```python
from build123d import *

# Parameters (mm, degrees)
F0_W         = 27.2
F0_H         = 2.5
F0_W_2       = 2.5
F0_H_2       = 33.7
F1_DEPTH     = 3
F2_R         = 2
F3_DEPTH     = 2
F4_W         = 2.5
F4_H         = 2.5
F5_DEPTH     = 1
F6_T1_DEPTH  = 9
F6_S5_W      = 2
F6_S5_H      = 2
F6_T6_DEPTH  = 2
F6_S11_W     = 2
F6_S11_H     = 2
F6_T12_DEPTH = 2
F6_S17_W     = 2
F6_S17_H     = 2
F6_T18_DEPTH = 2
F6_S23_W     = 2
F6_S23_H     = 2
F6_T24_DEPTH = 2


# Not quite as in the source:
# - a fillet or chamfer that OpenCascade refuses, or shapes differently, is made with other operations: its cross-section is extruded or revolved along the edge and cut away or added


with BuildPart() as f1:
    # F0 (on Top) → F1 (new body)
    with BuildSketch(Plane.XY):
        with Locations((0.1669520199, 18.5940534235)):
            Rectangle(F0_W, F0_H)
        with Locations((-14.6830479801, 0.4940534235)):
            Rectangle(F0_W_2, F0_H_2)
        with Locations((-14.6830479801, 18.5940534235)):
            Rectangle(F0_W_2, F0_H)
        with Locations((-14.6830479801, -17.6059465765)):
            Rectangle(F0_W_2, F0_H)
        with Locations((0.1669520199, -17.6059465765)):
            Rectangle(F0_W, F0_H)
        with Locations((15.0169520199, -17.6059465765)):
            Rectangle(F0_W_2, F0_H)
        with Locations((15.0169520199, 0.4940534235)):
            Rectangle(F0_W_2, F0_H_2)
        with Locations((15.0169520199, 18.5940534235)):
            Rectangle(F0_W_2, F0_H)
    extrude(amount=F1_DEPTH)

    # F2
    f2_edges = [f1.edges().sort_by_distance(p)[0] for p in [
        (16.266952, 0.494053, 3),
        (0.166952, 19.844053, 3),
        (-15.933048, 0.494053, 3),
        (0.166952, -18.855947, 3),
    ]]
    fillet(f2_edges, radius=F2_R)

    # F0 (on Top) → F3 (join)
    with BuildSketch(Plane.XY):
        with Locations((-14.6830479801, -17.6059465765)):
            Rectangle(F0_W_2, F0_H)
        with Locations((15.0169520199, -17.6059465765)):
            Rectangle(F0_W_2, F0_H)
        with Locations((15.0169520199, 18.5940534235)):
            Rectangle(F0_W_2, F0_H)
        with Locations((-14.6830479801, 18.5940534235)):
            Rectangle(F0_W_2, F0_H)
    extrude(amount=-F3_DEPTH)

    # F4 (on face) → F5 (join)
    with BuildSketch(Plane(origin=(0, 0, -2), x_dir=(1, 0, 0), z_dir=(0, 0, -1))):
        Polygon((-13.4330479801, -19.8440534235), (16.2669520199, -19.8440534235), (16.2669520199, 18.8559465765), (-15.9330479801, 18.8559465765), (-15.9330479801, -17.3440534235), (-13.4330479801, -17.3440534235), align=None)
        with Locations((-14.6830479801, -18.5940534235)):
            Rectangle(F4_W, F4_H)
    extrude(amount=F5_DEPTH)

    # F6: fillet of radius 2 on 4 edges, made by hand

    # F6_s2 → F6_t1 (cut)
    with BuildSketch(Plane.XY.offset(-8)):
        with BuildLine():
            ThreePointArc((16.2669520199, 17.8440534235), (15.6811655823, 19.2582669858), (14.2669520199, 19.8440534235))
            Line((14.2669520199, 19.8440534235), (16.2669520199, 19.8440534235))
            Line((16.2669520199, 19.8440534235), (16.2669520199, 17.8440534235))
        make_face()
        with BuildLine():
            ThreePointArc((16.2669520199, -16.8559465765), (15.6811655823, -18.2701601389), (14.2669520199, -18.8559465765))
            Line((14.2669520199, -18.8559465765), (16.2669520199, -18.8559465765))
            Line((16.2669520199, -18.8559465765), (16.2669520199, -16.8559465765))
        make_face()
        with BuildLine():
            ThreePointArc((-15.9330479801, -16.8559465765), (-15.3472615424, -18.2701601389), (-13.9330479801, -18.8559465765))
            Line((-13.9330479801, -18.8559465765), (-15.9330479801, -18.8559465765))
            Line((-15.9330479801, -18.8559465765), (-15.9330479801, -16.8559465765))
        make_face()
        with BuildLine():
            ThreePointArc((-15.9330479801, 17.8440534235), (-15.3472615424, 19.2582669858), (-13.9330479801, 19.8440534235))
            Line((-13.9330479801, 19.8440534235), (-15.9330479801, 19.8440534235))
            Line((-15.9330479801, 19.8440534235), (-15.9330479801, 17.8440534235))
        make_face()
    extrude(amount=F6_T1_DEPTH, mode=Mode.SUBTRACT)


with BuildPart() as f6_tool4:
    # F6_s5 → F6_t6 (new body)
    with BuildSketch(Plane.YZ.offset(-13.9330479801)):
        with Locations((18.8440534235, 2)):
            Rectangle(F6_S5_W, F6_S5_H)
    extrude(amount=-F6_T6_DEPTH)

    # F6_s7 → F6_t8 (revolve, cut)
    with BuildSketch(Plane(origin=(-13.9330479801, 17.8440534235, 1), x_dir=(0, -0.7071067812, -0.7071067812), z_dir=(0, 0.7071067812, -0.7071067812))):
        with BuildLine():
            ThreePointArc((0, -2), (2, 0), (0, 2))
            Line((0, 2), (0, -2))
        make_face()
    revolve(axis=Axis((-13.9330479801, 17.8440534235, 1), (-1, 0, 0)), mode=Mode.SUBTRACT)


with BuildPart() as f1_1:
    add(f1.part)

    # F6_t3: cut F6_tool4
    add(f6_tool4.part, mode=Mode.SUBTRACT)


with BuildPart() as f6_tool10:
    # F6_s11 → F6_t12 (new body)
    with BuildSketch(Plane.YZ.offset(-13.9330479801)):
        with Locations((-17.8559465765, 2)):
            Rectangle(F6_S11_W, F6_S11_H)
    extrude(amount=-F6_T12_DEPTH)

    # F6_s13 → F6_t14 (revolve, cut)
    with BuildSketch(Plane(origin=(-13.9330479801, -16.8559465765, 1), x_dir=(0, 0.7071067812, -0.7071067812), z_dir=(0, 0.7071067812, 0.7071067812))):
        with BuildLine():
            ThreePointArc((0, -2), (2, 0), (0, 2))
            Line((0, 2), (0, -2))
        make_face()
    revolve(axis=Axis((-13.9330479801, -16.8559465765, 1), (-1, 0, 0)), mode=Mode.SUBTRACT)


with BuildPart() as f1_2:
    add(f1_1.part)

    # F6_t9: cut F6_tool10
    add(f6_tool10.part, mode=Mode.SUBTRACT)


with BuildPart() as f6_tool16:
    # F6_s17 → F6_t18 (new body)
    with BuildSketch(Plane.YZ.offset(14.2669520199)):
        with Locations((-17.8559465765, 2)):
            Rectangle(F6_S17_W, F6_S17_H)
    extrude(amount=F6_T18_DEPTH)

    # F6_s19 → F6_t20 (revolve, cut)
    with BuildSketch(Plane(origin=(14.2669520199, -16.8559465765, 1), x_dir=(0, 0.7071067812, -0.7071067812), z_dir=(0, -0.7071067812, -0.7071067812))):
        with BuildLine():
            ThreePointArc((0, -2), (2, 0), (0, 2))
            Line((0, 2), (0, -2))
        make_face()
    revolve(axis=Axis((14.2669520199, -16.8559465765, 1), (1, 0, 0)), mode=Mode.SUBTRACT)


with BuildPart() as f1_3:
    add(f1_2.part)

    # F6_t15: cut F6_tool16
    add(f6_tool16.part, mode=Mode.SUBTRACT)


with BuildPart() as f6_tool22:
    # F6_s23 → F6_t24 (new body)
    with BuildSketch(Plane.YZ.offset(14.2669520199)):
        with Locations((18.8440534235, 2)):
            Rectangle(F6_S23_W, F6_S23_H)
    extrude(amount=F6_T24_DEPTH)

    # F6_s25 → F6_t26 (revolve, cut)
    with BuildSketch(Plane(origin=(14.2669520199, 17.8440534235, 1), x_dir=(0, -0.7071067812, -0.7071067812), z_dir=(0, -0.7071067812, 0.7071067812))):
        with BuildLine():
            ThreePointArc((0, -2), (2, 0), (0, 2))
            Line((0, 2), (0, -2))
        make_face()
    revolve(axis=Axis((14.2669520199, 17.8440534235, 1), (1, 0, 0)), mode=Mode.SUBTRACT)


with BuildPart() as f1_4:
    add(f1_3.part)

    # F6_t21: cut F6_tool22
    add(f6_tool22.part, mode=Mode.SUBTRACT)


solid = f1_4.part
```
Geometry check sheet. Reference: the model listing, model coordinates, mm. A direction names the side the tool comes from. Give positions to 0.01 mm unless a question says otherwise; leave off trailing zeros. Loops run counter-clockwise (first coordinate to the right, second up) from the corner with the lowest first, then second, coordinate; pieces in that order, holes last. Notation, with made-up numbers: M 62,-34.5 L 66,-34.5 A13 ccw 66,-26.5 Z; hole C 87.5,29 d1. An arc over 180 degrees is marked long. Write item = value, one per line. Start each with the question number.
1. Section check C-C, the plane x = -12. Enter the section's corners in (y, z).
2. Go/stop test with flat-tipped pins: P1, Ø1.5, axis at x = -9.5, y = -9.5, coming from the +Z side; P2, Ø0.9, axis at x = 3.5, z = 2, coming from the -Y side; P3, Ø0.6, axis at x = 15, z = -0.5, coming from the +Y side. Record where each tip stops, or that it passes through.
3. Section check D-D, the plane z = 2.25. Enter the section's corners in (x, y), plus the area to 3 significant figures.
4. Section check B-B, the plane y = 11.5. Enter the section's corners in (x, z), plus the area to 3 significant figures.
5. Section check A-A, the plane z = -0.85. Enter the section's corners in (x, y).
6. Draft check along Y on faces 4 (the face through (15, -16.356, -1)), 5 (the face through (13.767, -18, -1)), 6 (the face through (0.364, -18.286, 2.399)), 7 (the face through (-15, -16.356, -1)). Enter one of: +Y half, -Y half, draft (parallel to the pull), parting line (faces both ways), or undercut.
7. Thickness scan on probe 1 along Y at (x, z) = (-7, 1.1); probe 2 along X at (y, z) = (-13.5, 0.8); probe 3 along Z at (x, y) = (-14, -6). Record the ranges inside material, lowest first.
8. Tool access check on faces 1 (the face through (0, 0, -2)), 2 (the face through (15, 1, 0)), 3 (the face through (-13.433, 0, 1)). Record the directions out of +Z, -Z, +X, -X, +Y, -Y that give a thin tool (end or side, any length) a straight path to the whole face; none if there is none.
Values follow:
q1.outline = M -18.86,-3 L 19.84,-3 L 19.84,-2 L -18.86,-2 Z; M -18.86,0 L -16.36,0 L -16.36,3 L -16.86,3 A2 ccw -18.86,1 Z; M 17.34,0 L 19.84,0 L 19.84,1 A2 ccw 17.84,3 L 17.34,3 Z
q2.P1 = -2
q2.P2 = -18.78
q2.P3 = 19.8
q3.outline = M -15.49,-16.86 A1.56 ccw -13.93,-18.42 L 14.27,-18.42 A1.56 ccw 15.83,-16.86 L 15.83,17.84 A1.56 ccw 14.27,19.41 L -13.93,19.41 A1.56 ccw -15.49,17.84 Z; hole M -13.43,-16.36 L 13.77,-16.36 L 13.77,17.34 L -13.43,17.34 Z
q3.area = 266 mm^2
q4.outline = M -15.93,-3 L 16.27,-3 L 16.27,-2 L -15.93,-2 Z; M -15.93,0 L -13.43,0 L -13.43,3 L -13.93,3 A2 ccw -15.93,1 Z; M 13.77,0 L 16.27,0 L 16.27,1 A2 ccw 14.27,3 L 13.77,3 Z
q4.area = 45.5 mm^2
q5.outline = M -15.93,-16.86 A2 ccw -13.93,-18.86 L -13.43,-18.86 L -13.43,-16.36 L -15.93,-16.36 Z; M -15.93,17.34 L -13.43,17.34 L -13.43,19.84 L -13.93,19.84 A2 ccw -15.93,17.84 Z; M 13.77,-18.86 L 14.27,-18.86 A2 ccw 16.27,-16.86 L 16.27,-16.36 L 13.77,-16.36 Z; M 13.77,17.34 L 16.27,17.34 L 16.27,17.84 A2 ccw 14.27,19.84 L 13.77,19.84 Z
q6.face_4 = undercut
q6.face_5 = draft
q6.face_6 = -Y half
q6.face_7 = undercut
q7.probe_1 = -18.85 to -16.36, 17.34 to 19.84
q7.probe_2 = -15.93 to -13.43, 13.77 to 16.27
q7.probe_3 = -3 to -2, 0 to 3
q8.face_1 = none
q8.face_2 = +X, -X
q8.face_3 = +Z
